Geometry: final body of the model. Coordinates: model frame, mm. A direction names the side the tool comes from. Give positions to 0.01 mm unless a question says otherwise; leave off trailing zeros.
Autodesk Inventor part; units mm, degrees
ref_plane "C1_XY" through (0, 0, 0) normal (0, 0, 1) x (1, 0, 0)
ref_plane "C1_YZ" through (0, 0, 0) normal (1, 0, 0) x (0, 1, 0)
ref_plane "C1_ZX" through (0, 0, 0) normal (0, 1, 0) x (0, 0, 1)
sketch "Sketch_1" plane through (0, 0, 0) normal (0, 0, 1) x (1, 0, 0)
  line L0 (-10, -7) -> (-8, -7)
  line L1 (-8, -7) -> (-8, -4)
  line L2 (-8, -4) -> (-7.0607, -4)
  line L3 (-7.0607, -4) -> (-4, -7.0607)
  line L4 (-4, -7.0607) -> (-4, -9.4804)
  line L5 (-4, -9.4804) -> (-3.7, -10)
  line L6 (-3.7, -10) -> (-4, -10.5196)
  line L7 (-4, -10.5196) -> (-4, -12.9393)
  line L8 (-4, -12.9393) -> (-7.0607, -16)
  line L9 (-7.0607, -16) -> (-8, -16)
  line L10 (-8, -16) -> (-8, -13)
  line L11 (-8, -13) -> (-10, -13)
  line L12 (-10, -13) -> (-10, -19)
  arc A0 (-10, -19) -> (-9, -20) centre (-9, -19) ccw
  line L13 (-9, -20) -> (-3, -20)
  line L14 (-3, -20) -> (-3, -18)
  line L15 (-3, -18) -> (-6, -18)
  line L16 (-6, -18) -> (-6, -17.0607)
  line L17 (-6, -17.0607) -> (-2.9393, -14)
  line L18 (-2.9393, -14) -> (-0.5196, -14)
  line L19 (-0.5196, -14) -> (0, -13.7)
  line L20 (0, -13.7) -> (0.5196, -14)
  line L21 (0.5196, -14) -> (2.9393, -14)
  line L22 (2.9393, -14) -> (6, -17.0607)
  line L23 (6, -17.0607) -> (6, -18)
  line L24 (6, -18) -> (3, -18)
  line L25 (3, -18) -> (3, -20)
  line L26 (3, -20) -> (9, -20)
  arc A1 (9, -20) -> (10, -19) centre (9, -19) ccw
  line L27 (10, -19) -> (10, -13)
  line L28 (10, -13) -> (8, -13)
  line L29 (8, -13) -> (8, -16)
  line L30 (8, -16) -> (7.0607, -16)
  line L31 (7.0607, -16) -> (4, -12.9393)
  line L32 (4, -12.9393) -> (4, -10.5196)
  line L33 (4, -10.5196) -> (3.7, -10)
  line L34 (3.7, -10) -> (4, -9.4804)
  line L35 (4, -9.4804) -> (4, -7.0607)
  line L36 (4, -7.0607) -> (7.0607, -4)
  line L37 (7.0607, -4) -> (8, -4)
  line L38 (8, -4) -> (8, -7)
  line L39 (8, -7) -> (10, -7)
  line L40 (10, -7) -> (10, 7)
  line L41 (10, 7) -> (8, 7)
  line L42 (8, 7) -> (8, 4)
  line L43 (8, 4) -> (7.0607, 4)
  line L44 (7.0607, 4) -> (4, 7.0607)
  line L45 (4, 7.0607) -> (4, 9.4804)
  line L46 (4, 9.4804) -> (3.7, 10)
  line L47 (3.7, 10) -> (4, 10.5196)
  line L48 (4, 10.5196) -> (4, 12.9393)
  line L49 (4, 12.9393) -> (7.0607, 16)
  line L50 (7.0607, 16) -> (8, 16)
  line L51 (8, 16) -> (8, 13)
  line L52 (8, 13) -> (10, 13)
  line L53 (10, 13) -> (10, 19)
  arc A2 (10, 19) -> (9, 20) centre (9, 19) ccw
  line L54 (9, 20) -> (3, 20)
  line L55 (3, 20) -> (3, 18)
  line L56 (3, 18) -> (6, 18)
  line L57 (6, 18) -> (6, 17.0607)
  line L58 (6, 17.0607) -> (2.9393, 14)
  line L59 (2.9393, 14) -> (0.5196, 14)
  line L60 (0.5196, 14) -> (0, 13.7)
  line L61 (0, 13.7) -> (-0.5196, 14)
  line L62 (-0.5196, 14) -> (-2.9393, 14)
  line L63 (-2.9393, 14) -> (-6, 17.0607)
  line L64 (-6, 17.0607) -> (-6, 18)
  line L65 (-6, 18) -> (-3, 18)
  line L66 (-3, 18) -> (-3, 20)
  line L67 (-3, 20) -> (-9, 20)
  arc A3 (-9, 20) -> (-10, 19) centre (-9, 19) ccw
  line L68 (-10, 19) -> (-10, 13)
  line L69 (-10, 13) -> (-8, 13)
  line L70 (-8, 13) -> (-8, 16)
  line L71 (-8, 16) -> (-7.0607, 16)
  line L72 (-7.0607, 16) -> (-4, 12.9393)
  line L73 (-4, 12.9393) -> (-4, 10.5196)
  line L74 (-4, 10.5196) -> (-3.7, 10)
  line L75 (-3.7, 10) -> (-4, 9.4804)
  line L76 (-4, 9.4804) -> (-4, 7.0607)
  line L77 (-4, 7.0607) -> (-7.0607, 4)
  line L78 (-7.0607, 4) -> (-8, 4)
  line L79 (-8, 4) -> (-8, 7)
  line L80 (-8, 7) -> (-10, 7)
  line L81 (-10, 7) -> (-10, -7)
  line L82 (-8, 1.7) -> (-8, -1.7)
  arc A4 (-8, -1.7) -> (-7.7, -2) centre (-7.7, -1.7) ccw
  line L83 (-7.7, -2) -> (-7.0636, -2)
  arc A5 (-6.8515, -2.0879) -> (-7.0636, -2) centre (-7.0636, -2.3) ccw
  line L84 (-6.8515, -2.0879) -> (-2.9393, -6)
  line L85 (-2.9393, -6) -> (2.9393, -6)
  line L86 (2.9393, -6) -> (6.8515, -2.0879)
  arc A6 (7.0636, -2) -> (6.8515, -2.0879) centre (7.0636, -2.3) ccw
  line L87 (7.0636, -2) -> (7.7, -2)
  arc A7 (7.7, -2) -> (8, -1.7) centre (7.7, -1.7) ccw
  line L88 (8, -1.7) -> (8, 1.7)
  arc A8 (8, 1.7) -> (7.7, 2) centre (7.7, 1.7) ccw
  line L89 (7.7, 2) -> (7.0636, 2)
  arc A9 (6.8515, 2.0879) -> (7.0636, 2) centre (7.0636, 2.3) ccw
  line L90 (6.8515, 2.0879) -> (2.9393, 6)
  line L91 (2.9393, 6) -> (-2.9393, 6)
  line L92 (-2.9393, 6) -> (-6.8515, 2.0879)
  arc A10 (-7.0636, 2) -> (-6.8515, 2.0879) centre (-7.0636, 2.3) ccw
  line L93 (-7.0636, 2) -> (-7.7, 2)
  arc A11 (-7.7, 2) -> (-8, 1.7) centre (-7.7, 1.7) ccw
extrude "Extrusion1" add sketch "Sketch_1" against normal blind 300
sketch "Sketch2" plane through (0, 0, -300) normal (0, 0, -1) x (-1, 0, 0)
  point P0 (0, 10)
hole "Hole1" at (0, 10, -300) direction (0, 0, 1) diameter 4.2 depth 300
pattern_linear "Rectangular Pattern1" count 2 spacing 20 along (0, -1, 0) of "Hole1"
ref_plane "C1_XY" through (0, 0, 0) normal (0, 0, 1) x (1, 0, 0)
ref_plane "C1_YZ" through (0, 0, 0) normal (1, 0, 0) x (0, 1, 0)
ref_plane "C1_ZX" through (0, 0, 0) normal (0, 1, 0) x (0, 0, 1)
properties part number "HFSB5-2040-300"
Q1. Material intervals for probe 1 along Y at (x, z) = (0, -171.5); probe 2 along Y at (x, z) = (9.25, -40); probe 3 along Y at (x, z) = (7.75, -67), sorted ascending.
Q2. Pin query (flat end, axial travel): pin 1 Ø3 at (x, z) = (-0.5, -237) entering from -Y; pin 2 Ø0.6 at (x, z) = (9.5, -84) entering from +Y. Return the tip coordinate at first contact, or that it passes through.
Q3. Section query A-A, the plane z = -219. State how many separate pieces and enclosed holes the cut face has, and give its area (3 significant figures).
Q4. Mould query, pull axis X, two halves, no side actions, for faces 3 (the face through (-6, -20, -148)), 4 (the face through (0, -6, -148)), 5 (the face through (10, 16, -148)). Classes: +X half, -X half, draft (parallel to the pull), parting line (faces both ways), or undercut.
Q5. Reachability of faces 1 (the face through (-6, 20, -148)), 2 (the face through (0, 6, -148)) from +Z, -Z, +X, -X, +Y, -Y: full face, straight path, thin tool, end or side. Return the list, or none.
Resolved:
1. probe 1: y = -13.7 to -12.1, -7.9 to -6, 6 to 7.9, 12.1 to 13.7
1. probe 2: y = -19.97 to -13, -7 to 7, 13 to 19.97
1. probe 3: y = -20 to -16, -4 to -2, 2 to 4, 16 to 20
2. pin 1: stops at y = -14
2. pin 2: stops at y = 19.98
3. separate pieces: 1
3. enclosed holes: 3
3. area: 324 mm2
4. face 3: draft
4. face 4: undercut
4. face 5: +X half
5. face 1: +Z, -Z, +X, -X, +Y
5. face 2: +Z, -Z
